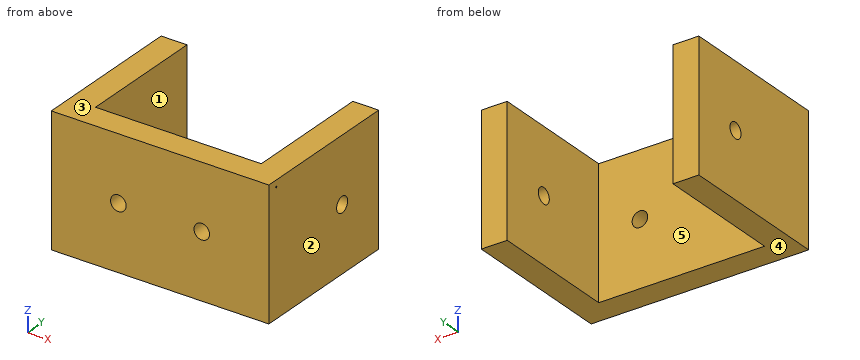
Autodesk Inventor part; units mm, degrees
ref_plane "YZ Plane" through (0, 0, 0) normal (1, 0, 0) x (0, 1, 0)
ref_plane "XZ Plane" through (0, 0, 0) normal (0, 1, 0) x (-1, 0, 0)
ref_plane "XY Plane" through (0, 0, 0) normal (0, 0, 1) x (1, 0, 0)
sketch "Sketch1" plane through (0, 0, 0) normal (0, 1, 0) x (-1, 0, 0)
  line L0 (21, 12.5) -> (-21, 12.5)
  line L1 (-21, 12.5) -> (-21, -12.5)
  line L2 (-21, -12.5) -> (21, -12.5)
  line L3 (21, -12.5) -> (21, 12.5)
  line L4 (21, 12.5) -> (-21, -12.5) construction
  line L5 (-21, 12.5) -> (21, -12.5) construction
  point P0 (0, 0)
  dimension "d0" = 42
  dimension "d1" = 25
extrude "Extrusion1" add sketch "Sketch1" along normal blind 5
sketch "Sketch5" plane through (-21, 0, -12.5) normal (-1, 0, 0) x (0, 0, 1)
  point P0 (12.5, 0)
sketch "Sketch6" plane through (21, 0, 12.5) normal (1, 0, 0) x (0, 0, -1)
  circle A0 centre (1.25, 2.0074) radius 0.15
  point P0 (12.5, 0)
  dimension "d11" = 0.3
extrude "Extrusion5" cut sketch "Sketch6" against normal blind 10
sketch "Sketch8" plane through (0, 5, 0) normal (0, 1, 0) x (1, 0, 0)
  line L0 (21, 12.5) -> (-21, 12.5)
  line L1 (-21, -12.5) -> (21, -12.5)
  line L2 (-21, 12.5) -> (-16, 12.5)
  line L3 (-16, 12.5) -> (-16, -12.5)
  line L4 (-16, -12.5) -> (-21, -12.5)
  line L5 (-21, -12.5) -> (-21, 12.5)
  point P0 (0, 0)
  dimension "d14" = 5
extrude "Extrusion6" add sketch "Sketch8" along normal blind 25
sketch "Sketch9" plane through (0, 5, 0) normal (0, 1, 0) x (1, 0, 0)
  line L0 (21, 12.5) -> (-21, 12.5)
  line L1 (-21, -12.5) -> (21, -12.5)
  line L2 (21, 12.5) -> (16, 12.5)
  line L3 (16, 12.5) -> (16, -12.5)
  line L4 (16, -12.5) -> (21, -12.5)
  line L5 (21, -12.5) -> (21, 12.5)
  point P0 (0, 0)
  point P1 (16, 12.5)
  dimension "d17" = 5
extrude "Extrusion7" add sketch "Sketch9" along normal blind 25
sketch "Sketch10" plane through (21, 0, 12.5) normal (1, 0, 0) x (0, 0, -1)
  circle A0 centre (12.5, 19.9992) radius 1.5
  point P0 (12.5, 0)
  dimension "d20" = 3
extrude "Extrusion8" cut sketch "Sketch10" against normal blind 100
sketch "Sketch11" plane through (0, 5, 0) normal (0, 1, 0) x (1, 0, 0)
  point P0 (0, 0)
sketch "Sketch12" plane through (0, 5, 0) normal (0, 1, 0) x (1, 0, 0)
  circle A0 centre (-8.051, 0) radius 1.5
  circle A1 centre (8.051, 0) radius 1.5
  point P0 (0, 0)
  dimension "d23" = 3
  dimension "d24" = 3
extrude "Extrusion9" cut sketch "Sketch12" against normal blind 10
properties part number "clamp"
Build history of the part. All positions in model axes, mm. Face numbers are marked on the shaded views. A direction names the side the tool comes from. Give positions to 0.01 mm unless a question says otherwise; leave off trailing zeros. Order: outer loops, then holes, each group sorted by start corner. A loop starts at its lowest first (then second) coordinate and runs counter-clockwise, first axis right, second up. Notation, with made-up numbers: M -20.5,9 L 5.5,9 A24 cw 5.5,34 Z; hole C 5.5,51.5 d10. An arc over 180 degrees is marked long. Return JSON: item names as keys, results as strings.
Q1. Flat gauge pins, fed straight in: pin 1 (2.5 mm diameter, centred on y = 20, z = 0, fed in from +X); pin 2 (5 mm diameter, centred on x = -8.051, z = 0, fed in from +Y). Where does each tip first touch, or does it go through?
Answer list:
{"pin 1": "passes through", "pin 2": "stops at y = 5"}
Q2. Band-saw the part on C-C (y = 20.75). Give the cut face in (x, z).
Answer list:
{"outline": "M -21,-12.5 L -16,-12.5 L -16,-1.3 L -21,-1.3 Z; M -21,1.3 L -16,1.3 L -16,12.5 L -21,12.5 Z; M 16,-12.5 L 21,-12.5 L 21,-1.3 L 16,-1.3 Z; M 16,1.3 L 21,1.3 L 21,12.5 L 16,12.5 Z"}
Q3. Two-plate mould, pull along X, no slides. Class the marked faces 1, 2 and 3: pulls with the +X half, pulls with the -X half, needs draft (parallel to the pull), parting line crosses it, or undercut.
Answer list:
{"face 1": "undercut", "face 2": "pulls with the +X half", "face 3": "needs draft"}
Q4. Band-saw the part on B-B (y = 24). Give the cut face in (x, z), then the cut area to 3 significant figures.
Answer list:
{"outline": "M -21,-12.5 L -16,-12.5 L -16,12.5 L -21,12.5 Z; M 16,-12.5 L 21,-12.5 L 21,12.5 L 16,12.5 Z", "area": "250 mm^2"}
Q5. Band-saw the part on A-A (z = 0). Give the cut face in (x, y).
Answer list:
{"outline": "M -21,0 L -9.55,0 L -9.55,5 L -16,5 L -16,18.5 L -21,18.5 Z; M -21,21.5 L -16,21.5 L -16,30 L -21,30 Z; M -6.55,0 L 6.55,0 L 6.55,5 L -6.55,5 Z; M 9.55,0 L 21,0 L 21,18.5 L 16,18.5 L 16,5 L 9.55,5 Z; M 16,21.5 L 21,21.5 L 21,30 L 16,30 Z"}
Q6. 3-axis set-ups, long thin cutter, end or side, ignore diameter. For the marked faces 4 and 5: which of +Z, -Z, +X, -X, +Y, -Y reach the whole face in a straight line?
Answer list:
{"face 4": "-Z, +X, -X, +Y, -Y", "face 5": "+Z, -Z, +Y"}
Q7. Band-saw the part on D-D (x = 13). Give the cut face in (y, z), then the cut area to 3 significant figures.
Answer list:
{"outline": "M 0,-12.5 L 5,-12.5 L 5,12.5 L 0,12.5 Z; hole C 2.01,11.25 d0.3", "area": "125 mm^2"}
Q8. Wall check: probe 1 along X at (y, z) = (2.95, 0); probe 2 along X at (y, z) = (13.25, -7.25); probe 3 along Y at (x, z) = (17.5, 11.25). Give the ranges that are in metal, low to high. Write a range as from..to.
Answer list:
{"probe 1": "x = -21..-9.55, -6.55..6.55, 9.55..21", "probe 2": "x = -21..-16, 16..21", "probe 3": "y = 0..1.86, 2.16..30"}
